from build123d import *

# Parameters (mm, degrees)
F0_W          = 60
F0_H          = 60
F1_DEPTH      = 30
F6_DEPTH      = 15
F8_DEPTH      = 14.001
F8_DEPTH_BACK = 14.001
F9_DEPTH      = 30.001
F19_DEPTH     = 60


with BuildPart() as f1:
    # F0 (on Top) → F1 (new body)
    with BuildSketch(Plane.XY):
        Rectangle(F0_W, F0_H)
    extrude(amount=F1_DEPTH)

    # F2 (on face) → F5 section 0
    with BuildSketch(Plane.XY.offset(30)):
        Polygon((30, 0), (0, 30), (-30, 0), (0, -30), align=None)
    # F4 (on offset) → F5 section 1
    with BuildSketch(Plane.XY.offset(70)):
        Polygon((14, 0), (0, 14), (-14, 0), (0, -14), align=None)
    loft()

    # F6 (add): a face of the model
    f6_faces = [f1.faces().sort_by_distance(p)[0] for p in [
        (0, 0, 70),
    ]]
    extrude(f6_faces, amount=F6_DEPTH)

    # F7 (on Right) → F8 (cut, two sides)
    with BuildSketch(Plane.YZ) as f8_sk:
        Polygon((14, 85), (0, 85), (14, 70), align=None)
        Polygon((0, 85), (-14, 85), (-14, 70), align=None)
    extrude(amount=-F8_DEPTH, mode=Mode.SUBTRACT)
    extrude(f8_sk.sketch, amount=F8_DEPTH_BACK, mode=Mode.SUBTRACT)

    # F9 (cut, through all): a face of the model
    f9_faces = [f1.faces().sort_by_distance(p)[0] for p in [
        (20, -20, 30),
    ]]
    extrude(f9_faces, amount=-F9_DEPTH, mode=Mode.SUBTRACT)

    # F13 (on offset) → F17 section 0
    with BuildSketch(Plane.YZ.offset(-14)):
        Polygon((14, -5), (14, 0), (14, 30), (-14, 15), (-14, 0), (-14, -5), align=None)
    # F11 (on offset) → F17 section 1
    with BuildSketch(Plane.YZ.offset(14)):
        Polygon((14, 15), (-14, 0), (-14, -5), (14, -5), (14, 0), align=None)
    loft(mode=Mode.SUBTRACT)

    # F18 (on face) → F19 (cut, through all)
    with BuildSketch(Plane.YZ.offset(30)):
        Polygon((14, 0), (14, 15), (0, 7.5), (0, 0), align=None)
        Polygon((0, 0), (0, 7.5), (-14, 0), align=None)
    extrude(amount=-F19_DEPTH, mode=Mode.SUBTRACT)


solid = f1.part
Design review of the part built by this model. Coordinates are the model's own, in mm. A direction names the side the tool comes from. Give positions to 0.01 mm unless a question says otherwise; leave off trailing zeros. Loops run counter-clockwise (first coordinate to the right, second up) from the corner with the lowest first, then second, coordinate; pieces in that order, holes last. Notation, with made-up numbers: (76.5, -32) - (95.5, -32) arc R6 cw to (95.5, -25) - close; hole circle Ø6 at (38, 81.5). An arc over 180 degrees is marked (long way). Write item = value, one per line.
1) Clearance check with flat-ended pins moving along their axes: pin 1 Ø24 at (x, y) = (-18.5, 9.5) entering from +Z; pin 2 Ø3 at (y, z) = (1, 59) entering from +X; pin 3 Ø6 at (x, z) = (-10.5, 42) entering from -Y; pin 4 Ø6 at (x, z) = (-11, 65.5) entering from +Y. State where each tip first meets the part, or that it passes through.
Result sheet:
pin_1 = 85
pin_2 = 18.85
pin_3 = -17.93
pin_4 = 8.03
2) To check wall thickness, follow line 1 (Z direction, x = -8.5, y = 27); line 2 (Y direction, x = 15.5, z = 14); line 3 (Y direction, x = 22, z = 12.5). State the ranges of each line that lie inside material, in increasing order.
Result sheet:
line_1 = 0 to 30
line_2 = -14.5 to 12.13, 14 to 30
line_3 = -8 to 9.33, 14 to 30
3) Tool access review of faces 5 (the face through (-9, -5, 76)), 6 (the face through (20.334, 3.307, 9.272)), 7 (the face through (21, 22, 30)), 8 (the face through (10, -4, 74)), 9 (the face through (-19, 19, 30)): name each direction out of +Z, -Z, +X, -X, +Y, -Y from which nothing blocks a thin tool from reaching the whole face with its end or side.
Result sheet:
face_5 = +Z, -X, -Y
face_6 = -Z, +X, -X
face_7 = +Z, +X, +Y
face_8 = +Z, +X, -Y
face_9 = +Z, -X, +Y
4) Draft analysis for pull direction Y (two halves, no side actions). For faces 1 (the face through (9, 5, 76)), 2 (the face through (-22, -21, 30)), 3 (the face through (-21.888, 0.196, 7.605)), 4 (the face through (-15, -30, 15)), state which applies: +Y half, -Y half, draft (parallel to the pull), parting line (faces both ways), or undercut.
Result sheet:
face_1 = +Y half
face_2 = draft
face_3 = undercut
face_4 = -Y half
5) Take a section at A-A on z = 72.5. State the section outline as (x, y) points, and give its area (3 significant figures).
Result sheet:
outline = (-14, 0) - (-2.33, -11.67) - (2.33, -11.67) - (14, 0) - (2.33, 11.67) - (-2.33, 11.67) - close
area = 381 mm2
